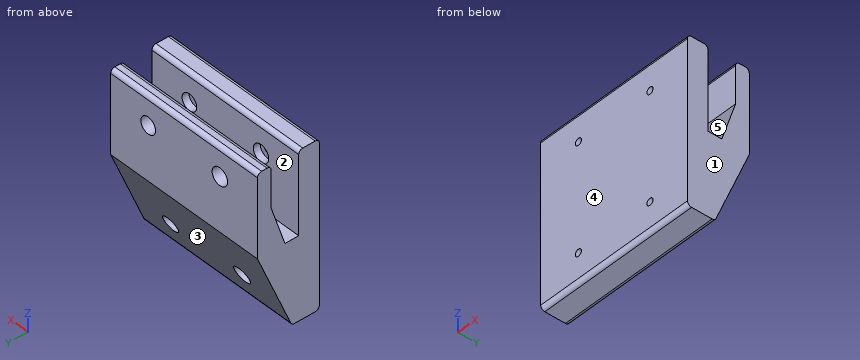
```python
from build123d import *

# Parameters (mm, degrees)
F1_DEPTH = 120
F2_R     = 2.5
F3_DEPTH = 45.001
F4_R     = 6
F4_R_2   = 6.300335
F5_DEPTH = 50.546
F6_DEPTH = 5
F7_R     = 3


with BuildPart() as f1:
    # F0 (on Right) → F1 (new body)
    with BuildSketch(Plane.YZ):
        Polygon((0, 60), (0, 0), (0, -60), (20, -60), (45, 0), (45, 60), (35, 60), (35, 30.086774), (25, 0), (15, 0), (15, 60), align=None)
    extrude(amount=F1_DEPTH)

    # F2 (on face) → F3 (cut, through all)
    with BuildSketch(Plane.XZ):
        with Locations((89.356575, 39.11762)):
            Circle(F2_R)
        with Locations((30.790308, 38.970736)):
            Circle(F2_R)
        with Locations((30.790308, -38.970736)):
            Circle(F2_R)
        with Locations((89.356575, -38.970736)):
            Circle(F2_R)
    extrude(amount=-F3_DEPTH, mode=Mode.SUBTRACT)

    # F4 (on face) → F5 (cut)
    with BuildSketch(Plane(origin=(0, 15, 0), x_dir=(-1, 0, 0), z_dir=(0, 1, 0))):
        with Locations((-89.356575, 39.11762)):
            Circle(F4_R)
        with Locations((-30.790308, 38.970736)):
            Circle(F4_R_2)
        with Locations((-89.356575, -39.11762)):
            Circle(F4_R)
        with Locations((-30.790308, -38.970736)):
            Circle(F4_R_2)
    extrude(amount=F5_DEPTH, mode=Mode.SUBTRACT)

    # F4 (on face) → F6 (cut)
    with BuildSketch(Plane(origin=(0, 15, 0), x_dir=(-1, 0, 0), z_dir=(0, 1, 0))):
        with Locations((-89.356575, 39.11762)):
            Circle(F4_R)
        with Locations((-30.790308, 38.970736)):
            Circle(F4_R_2)
        with Locations((-89.356575, -39.11762)):
            Circle(F4_R)
        with Locations((-30.790308, -38.970736)):
            Circle(F4_R_2)
    extrude(amount=-F6_DEPTH, mode=Mode.SUBTRACT)

    # F7
    f7_edges = [f1.edges().sort_by_distance(p)[0] for p in [
        (60, 0, 60),
        (60, 15, 60),
        (60, 35, 60),
        (60, 45, 60),
        (60, 0, -60),
        (60, 20, -60),
    ]]
    fillet(f7_edges, radius=F7_R)


solid = f1.part
```
Geometry check sheet. Reference: the model listing, model coordinates, mm. Face numbers are marked on the shaded views. A direction names the side the tool comes from. Give positions to 0.01 mm unless a question says otherwise; leave off trailing zeros. Order: outer loops, then holes, each group sorted by start corner. A loop starts at its lowest first (then second) coordinate and runs counter-clockwise, first axis right, second up. Notation, with made-up numbers: (52.5, 56.25) - (95.5, 56.25) arc R13 ccw to (95.5, 64.25) - close; hole circle Ø10 at (72, 62). An arc over 180 degrees is marked (long way). Answer in a Markdown table with one row per item. Add a question column.
Q1. Cross-section at A-A, the plane x = 35.5. Enter the section's corners in (y, z), then the cut area to 3 significant figures.
Q2. Cross-section at C-C, the plane x = 9. Enter the section's corners in (y, z).
Q3. Cross-section at B-B, the plane y = 13.5. Enter the section's corners in (x, z), then the cut area to 3 significant figures.
Q4. Cross-section at D-D, the plane y = 22.5. Enter the section's corners in (x, z).
Q5. Gauge pin test, flat ends, axial feed: pin 1 (9.5 mm diameter, centred on x = 88.5, z = -38.5, fed in from +Y); pin 2 (15.5 mm diameter, centred on x = 89.36, z = -39.12, fed in from +Y); pin 3 (3 mm diameter, centred on x = 89.36, z = -38.97, fed in from -Y); pin 4 (12 mm diameter, centred on x = 44, y = 37.5, fed in from -Z). Record the tip position at first contact, or that the pin passes through.
Q6. Tool access check on the marked faces 4 and 5. Record the directions out of +Z, -Z, +X, -X, +Y, -Y that give a thin tool (end or side, any length) a straight path to the whole face; none if there is none.
Q7. Mould release check, pull along Y, two halves, no side actions. Record for the marked faces 1, 2 and 3: pulls with the +Y half, pulls with the -Y half, needs draft (parallel to the pull), parting line crosses it, or undercut.
Q8. Material ranges on probe 1 along Z at (x, y) = (90, 11.5); probe 2 along Y at (x, z) = (47, 23); probe 3 along Y at (x, z) = (111, 49.5), recorded low to high. Write a range as from..to.
Check values:
| question | item | result |
|---|---|---|
| 1 | outline | (0, -57) arc R3 ccw to (3, -60) - (18, -60) arc R3 ccw to (20.77, -58.15) - (27.02, -43.16) - (10, -43.16) - (10, -34.79) - (30.51, -34.79) - (45, 0) - (45, 34.79) - (35, 34.79) - (35, 30.09) - (25, 0) - (15, 0) - (15, 34.79) - (10, 34.79) - (10, 43.16) - (15, 43.16) - (15, 57) arc R3 ccw to (12, 60) - (3, 60) arc R3 ccw to (0, 57) - close; (35, 43.16) - (45, 43.16) - (45, 57) arc R3 ccw to (42, 60) - (38, 60) arc R3 ccw to (35, 57) - close |
| 1 | area | 3,310 mm^2 |
| 2 | outline | (0, -57) arc R3 ccw to (3, -60) - (18, -60) arc R3 ccw to (20.77, -58.15) - (45, 0) - (45, 57) arc R3 ccw to (42, 60) - (38, 60) arc R3 ccw to (35, 57) - (35, 30.09) - (25, 0) - (15, 0) - (15, 57) arc R3 ccw to (12, 60) - (3, 60) arc R3 ccw to (0, 57) - close |
| 3 | outline | (0, -60) - (120, -60) - (120, 59.6) - (0, 59.6) - close; hole circle Ø12.6 at (30.79, -38.97); hole circle Ø12.6 at (30.79, 38.97); hole circle Ø12 at (89.36, -39.12); hole circle Ø12 at (89.36, 39.12) |
| 3 | area | 13,900 mm^2 |
| 4 | outline | (0, -54) - (120, -54) - (120, 0) - (0, 0) - close; hole circle Ø12.6 at (30.79, -38.97); hole circle Ø12 at (89.36, -39.12) |
| 5 | pin 1 | stops at y = 10 |
| 5 | pin 2 | stops at y = 31.93 |
| 5 | pin 3 | passes through |
| 5 | pin 4 | stops at z = -32.4 |
| 6 | face 4 | +Z, -Z, +X, -X, -Y |
| 6 | face 5 | +Z, +X, -X |
| 7 | face 1 | needs draft |
| 7 | face 2 | undercut |
| 7 | face 3 | pulls with the +Y half |
| 8 | probe 1 | z = -60..-45.08, -33.15..33.15, 45.08..60 |
| 8 | probe 2 | y = 0..15, 32.64..45 |
| 8 | probe 3 | y = 0..15, 35..45 |
